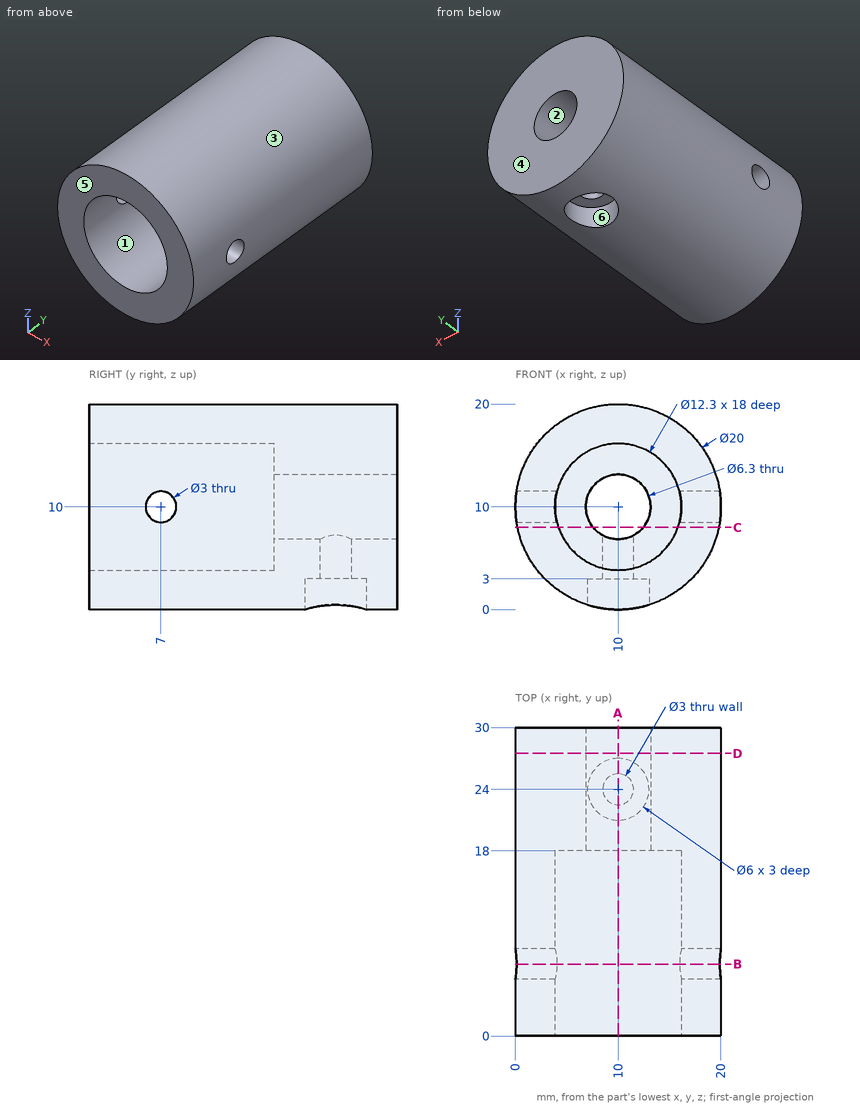
Design review of the part shown in the three views and the two pictorial views. Dimensions are in mm from the part's minimum x, y and z. A direction names the side the tool comes from. Coordinates: 2 decimals unless noted, no trailing zeros. Write each loop counter-clockwise with the first axis right and the second up, starting at its lowest first coordinate (ties: lowest second). Pieces come first, ordered by that corner, then holes. Notation, with made-up numbers: (44.5, 72.5) -> (103.5, 72.5) arc R27 ccw to (103.5, 103.5) -> close; hole circle Ø11 at (-35, 20). An arc over 180 degrees is marked (long way). Answer in a Markdown table with one row per item.
1. For the marked faces 5 and 6, list the 3-axis set-ups (+Z, -Z, +X, -X, +Y, -Y) from which the entire face can be reached by the end or side of a thin tool; tool diameter is ignored.
Answers below:
| item | result |
|---|---|
| face 5 | +Z, -Z, +X, -X, -Y |
| face 6 | -Z |
2. Clearance check with flat-ended pins moving along their axes: pin 1 Ø10 at (x, z) = (10, 10) entering from +Y; pin 2 Ø2 at (y, z) = (17.5, 13) entering from -X; pin 3 Ø2.5 at (y, z) = (7, 10) entering from +X; pin 4 Ø5 at (x, y) = (9, 24) entering from -Z. State where each tip first meets the part, or that it passes through.
Answers below:
| item | result |
|---|---|
| pin 1 | stops at y = 30 |
| pin 2 | stops at x = 0.2 |
| pin 3 | passes through |
| pin 4 | stops at z = 0.18 |
3. We need section B-B, the plane y = 7. State the section outline as (x, z) points.
Answers below:
| item | result |
|---|---|
| outline | (0.11, 8.5) arc R10 ccw to (19.89, 8.5) -> (15.96, 8.5) arc R6.15 cw to (4.04, 8.5) -> close; (0.11, 11.5) -> (4.04, 11.5) arc R6.15 cw to (15.96, 11.5) -> (19.89, 11.5) arc R10 ccw to start |
4. We need section D-D, the plane y = 27.5. State the section outline as (x, z) points.
Answers below:
| item | result |
|---|---|
| outline | circle Ø20 at (10, 10); hole circle Ø6.3 at (10, 10) |
5. Wall thickness on probe 1 along Y at (x, z) = (1.5, 10); probe 2 along Y at (x, z) = (6.75, 13.5); probe 3 along X at (y, z) = (24, 1.8): over which ranges is each line inside the solid? List them lowest first. Write a range as [from, to].
Answers below:
| item | result |
|---|---|
| probe 1 | y = [0, 5.5], [8.5, 30] |
| probe 2 | y = [18, 30] |
| probe 3 | x = [4.28, 7], [13, 15.72] |
6. We need section C-C, the plane z = 8. State the section outline as (x, y) points.
Answers below:
| item | result |
|---|---|
| outline | (0.2, 0) -> (4.18, 0) -> (4.18, 18) -> (7.57, 18) -> (7.57, 30) -> (0.2, 30) -> close; (12.43, 18) -> (15.82, 18) -> (15.82, 0) -> (19.8, 0) -> (19.8, 30) -> (12.43, 30) -> close |
7. Draft analysis for pull direction Z (two halves, no side actions). For the marked faces 1, 2, 3 and 4, state which applies: +Z half, -Z half, draft (parallel to the pull), parting line (faces both ways), or undercut.
Answers below:
| item | result |
|---|---|
| face 1 | undercut |
| face 2 | undercut |
| face 3 | parting line |
| face 4 | draft |
8. We need section A-A, the plane x = 10. State the section outline as (y, z) points.
Answers below:
| item | result |
|---|---|
| outline | (0, 0) -> (21, 0) -> (21, 3) -> (22.5, 3) -> (22.5, 6.85) -> (18, 6.85) -> (18, 3.85) -> (0, 3.85) -> close; (0, 16.15) -> (18, 16.15) -> (18, 13.15) -> (30, 13.15) -> (30, 20) -> (0, 20) -> close; (25.5, 3) -> (27, 3) -> (27, 0) -> (30, 0) -> (30, 6.85) -> (25.5, 6.85) -> close |
